from build123d import *

# Parameters (mm, degrees)
SKETCH1_W               = 50.8
SKETCH1_H               = 571.5
BOSS_EXTRUDE1_DEPTH     = 12.7
SHELL1_T                = -1.5875
CUT_EXTRUDE1_DEPTH      = 288.157643987
CUT_EXTRUDE1_DEPTH_BACK = 288.157643987
SKETCH2_R               = 2.4892
CUT_EXTRUDE2_DEPTH      = 288.157643987
CUT_EXTRUDE2_DEPTH_BACK = 288.157643987
SKETCH3_R               = 2.4892
SKETCH4_W               = 31.75
SKETCH4_H               = 26.9875
CUT_EXTRUDE3_DEPTH      = 288.157643987
FILLET1_R               = 3.175
FILLET1_OF_MIRROR1_R    = 3.175
FILLET2_R               = 3.175


with BuildPart() as part:
    # Sketch1 → Boss-Extrude1 (new, symmetric)
    with BuildSketch(Plane.XY):
        Rectangle(SKETCH1_W, SKETCH1_H)
    extrude(amount=BOSS_EXTRUDE1_DEPTH, both=True)

    # Shell1
    shell1_openings = [part.faces().sort_by_distance(p)[0] for p in [
        (0, -285.75, 0),
        (0, 285.75, 0),
    ]]
    offset(amount=SHELL1_T, openings=shell1_openings, kind=Kind.INTERSECTION)

    # Sketch2 → Cut-Extrude1 (cut, two sides: drawn at the far end of the back side and taken through both)
    with BuildSketch(Plane.XY.offset(-CUT_EXTRUDE1_DEPTH_BACK)):
        with Locations((-12.7, -273.05)):
            Circle(SKETCH2_R)
        with Locations((12.7, -273.05)):
            Circle(SKETCH2_R)
        with Locations(Location((12.7, 273.05, 0), (0, 0, 180))):
            Circle(SKETCH2_R)
        with Locations(Location((-12.7, 273.05, 0), (0, 0, 180))):
            Circle(SKETCH2_R)
    extrude(amount=CUT_EXTRUDE1_DEPTH + CUT_EXTRUDE1_DEPTH_BACK, mode=Mode.SUBTRACT)

    # Sketch3 → Cut-Extrude2 (cut, two sides: drawn at the far end of the back side and taken through both)
    with BuildSketch(Plane(origin=(0, 0, 0), x_dir=(0, 0, -1), z_dir=(1, 0, 0)).offset(-CUT_EXTRUDE2_DEPTH_BACK)):
        with Locations((0, -273.05)):
            Circle(SKETCH3_R)
        with Locations((0, 273.05)):
            Circle(SKETCH3_R)
    extrude(amount=CUT_EXTRUDE2_DEPTH + CUT_EXTRUDE2_DEPTH_BACK, mode=Mode.SUBTRACT)

    # Sketch4 → Cut-Extrude3 (cut, symmetric)
    with BuildSketch(Plane.XY):
        with Locations((0, 241.3)):
            Rectangle(SKETCH4_W, SKETCH4_H)
    cut_extrude3 = extrude(amount=CUT_EXTRUDE3_DEPTH, both=True, mode=Mode.SUBTRACT)

    # Fillet1
    fillet1_edges = [part.edges().sort_by_distance(p)[0] for p in [
        (-15.875, 227.80625, -11.90625),
        (-15.875, 254.79375, -11.90625),
        (15.875, 254.79375, -11.90625),
        (15.875, 227.80625, -11.90625),
    ]]
    fillet(fillet1_edges, radius=FILLET1_R)

    # Mirror1: Cut-Extrude3 across plane
    add(cut_extrude3.mirror(Plane.ZX), mode=Mode.SUBTRACT)

    # Fillet1 of Mirror1
    fillet1_of_mirror1_edges = [part.edges().sort_by_distance(p)[0] for p in [
        (-15.875, -227.80625, -11.90625),
        (-15.875, -254.79375, -11.90625),
        (15.875, -254.79375, -11.90625),
        (15.875, -227.80625, -11.90625),
    ]]
    fillet(fillet1_of_mirror1_edges, radius=FILLET1_OF_MIRROR1_R)

    # Fillet2
    fillet2_edges = [part.edges().sort_by_distance(p)[0] for p in [
        (-15.875, -254.79375, 11.90625),
        (-15.875, -227.80625, 11.90625),
        (15.875, -227.80625, 11.90625),
        (15.875, -254.79375, 11.90625),
        (-15.875, 227.80625, 11.90625),
        (-15.875, 254.79375, 11.90625),
        (15.875, 254.79375, 11.90625),
        (15.875, 227.80625, 11.90625),
    ]]
    fillet(fillet2_edges, radius=FILLET2_R)


solid = part.part
Read the model definition and answer for the solid it produces. Units are mm, in the model's axes. A direction names the side the tool comes from. Round coordinates to 2 decimals unless told otherwise and drop trailing zeros. Write each loop counter-clockwise with the first axis right and the second up, starting at its lowest first coordinate (ties: lowest second). Pieces come first, ordered by that corner, then holes.
1. The part is cut by section A-A, the plane x = 2. Determine the outline of the cut face in (y, z), then the cut area to 3 significant figures.
2. Determine the mould class of faces 3 (the face through (0, 4, 12.7)), 4 (the face through (0, 4, 11.112)), 5 (the face through (0, 285.75, -12)) for opening direction Z: pulls with the +Z half, pulls with the -Z half, needs draft (parallel to the pull), parting line crosses it, or undercut.
3. Straight lines are drawn through the part: L1, parallel to X at y = -273.05, z = -11.8; L2, parallel to Y at x = -12.7, z = -11.5; L3, parallel to X at y = -88, z = -10.25. For each, find the intervals that lie inside material, in ascending order.
4. Which of the six approach directions +Z, -Z, +X, -X, +Y, -Y give full straight-line access (tool end or side, diameter ignored) to faces 1 (the face through (-23.812, -4, 0)), 2 (the face through (0, -285.75, -12))?
5. The part is cut by section B-B, the plane y = 142.5. Determine the outline of the cut face in (x, z), then the cut area to 3 significant figures.
Values:
1. outline: (-285.75, -12.7) - (-254.79, -12.7) - (-254.79, -11.11) - (-285.75, -11.11) - close; (-285.75, 11.11) - (-254.79, 11.11) - (-254.79, 12.7) - (-285.75, 12.7) - close; (-227.81, -12.7) - (227.81, -12.7) - (227.81, -11.11) - (-227.81, -11.11) - close; (-227.81, 11.11) - (227.81, 11.11) - (227.81, 12.7) - (-227.81, 12.7) - close; (254.79, -12.7) - (285.75, -12.7) - (285.75, -11.11) - (254.79, -11.11) - close; (254.79, 11.11) - (285.75, 11.11) - (285.75, 12.7) - (254.79, 12.7) - close
1. area: 1,640 mm2
2. face 3: pulls with the +Z half
2. face 4: undercut
2. face 5: needs draft
3. L1: x = -25.4 to -15.19, -10.21 to 10.21, 15.19 to 25.4
3. L2: y = -285.75 to -275.54, -270.56 to -254.79, -227.81 to 227.81, 254.79 to 270.56, 275.54 to 285.75
3. L3: x = -25.4 to -23.81, 23.81 to 25.4
4. face 1: +Y, -Y
4. face 2: +Z, -Z, +X, -X, -Y
5. outline: (-25.4, -12.7) - (25.4, -12.7) - (25.4, 12.7) - (-25.4, 12.7) - close; hole (-23.81, -11.11) - (23.81, -11.11) - (23.81, 11.11) - (-23.81, 11.11) - close
5. area: 232 mm2
